```python
from build123d import *

# Parameters (mm, degrees)
CUT_EXTRUDE1_DEPTH = 2


# Read off the part's stored shape, not the designer's step: M6x1.0 Machine Threads Stud1
with BuildPart() as part:
    # Sketch1 → Revolve1 (revolve)
    with BuildSketch(Plane.XY, mode=Mode.PRIVATE) as revolve1_sk:
        with BuildLine():
            Line((0, -16.59536458), (0, 2.796940265))
            Line((0, 2.796940265), (3, 2.796940265))
            ThreePointArc((3, 2.796940265), (6, -2.399212157), (3, -7.59536458))
            Line((3, -7.59536458), (3, -16.59536458))
            Line((3, -16.59536458), (0, -16.59536458))
        make_face()
    revolve(revolve1_sk.sketch.rotate(Axis((0, -16.59536458, 0), (0, 1, 0)), 90), axis=Axis((0, -16.59536458, 0), (0, 1, 0)))

    # Sketch4 → Cut-Extrude1 (cut)
    with BuildSketch(Plane(origin=(0, 2.796940265, 0), x_dir=(1, 0, 0), z_dir=(0, 1, 0))):
        Polygon((-2.05, 0), (-1.025, -1.775352078), (1.025, -1.775352078), (2.05, 0), (1.025, 1.775352078), (-1.025, 1.775352078), align=None)
    extrude(amount=-CUT_EXTRUDE1_DEPTH, mode=Mode.SUBTRACT)

    # M6x1.0 Machine Threads Stud1 outline → M6x1.0 Machine Threads Stud1 (revolve, cut)
    with BuildSketch(Plane.XY):
        Polygon((3, -16.04086458), (2.4455, -16.59536458), (3, -16.59536458), align=None)
    revolve(axis=Axis((0, 0, 0), (0, 1, 0)), mode=Mode.SUBTRACT)


solid = part.part
```
Work out the finished part from the listing and answer in its coordinate system (mm). A direction names the side the tool comes from. Coordinates: 2 decimals unless noted, no trailing zeros. Loops run counter-clockwise (first coordinate to the right, second up) from the corner with the lowest first, then second, coordinate; pieces in that order, holes last. Notation, with made-up numbers: (27, 18.5) - (31, 18.5) arc R19 ccw to (31, 38.5) - close; hole circle Ø10 at (40, 87). An arc over 180 degrees is marked (long way). Use a Markdown table: item, result.
Item 1: Find section C-C, the plane y = -13.25. Determine the outline of the cut face in (x, z).
Evaluation:
| item | result |
|---|---|
| outline | circle Ø6 at (0, 0) |
Item 2: Find section D-D, the plane z = 4. Determine the outline of the cut face in (x, y), and give its area (3 significant figures).
Evaluation:
| item | result |
|---|---|
| outline | circle Ø8.94 at (0, -2.4) |
| area | 62.8 mm2 |
Item 3: Given pin 1 Ø0.6 at (x, y) = (0.5, 2) entering from -Z; pin 2 Ø2 at (y, z) = (-14.5, 0) entering from -X; pin 3 Ø1 at (y, z) = (-10, 0.5) entering from +X, each flat-ended and moving along its own axis, determine where each tip first touches the part or whether it passes through.
Evaluation:
| item | result |
|---|---|
| pin 1 | stops at z = -4.35 |
| pin 2 | stops at x = -3 |
| pin 3 | stops at x = 3 |
Item 4: Find section A-A, the plane x = 0. Determine the outline of the cut face in (y, z).
Evaluation:
| item | result |
|---|---|
| outline | (-16.6, -2.45) - (-16.04, -3) - (-7.6, -3) arc R6 ccw to (2.8, -3) - (2.8, -1.78) - (0.8, -1.78) - (0.8, 1.78) - (2.8, 1.78) - (2.8, 3) arc R6 ccw to (-7.6, 3) - (-16.04, 3) - (-16.6, 2.45) - close |
Item 5: Find section B-B, the plane y = 1.25. Determine the outline of the cut face in (x, z) (3 decimals), and give its area (3 significant figures).
Evaluation:
| item | result |
|---|---|
| outline | circle Ø9.525 at (0, 0); hole (-2.05, 0) - (-1.025, -1.775) - (1.025, -1.775) - (2.05, 0) - (1.025, 1.775) - (-1.025, 1.775) - close |
| area | 60.3 mm2 |
Item 6: Consider probe 1 along Y at (x, z) = (-0.75, 1.5); probe 2 along X at (y, z) = (-3, -0.5); probe 3 along X at (y, z) = (-7.5, 1). Determine where each line is inside the solid, lowest interval first. Write a range as from..to.
Evaluation:
| item | result |
|---|---|
| probe 1 | y = -16.6..0.8 |
| probe 2 | x = -5.95..5.95 |
| probe 3 | x = -3..3 |
Item 7: For faces 1 (the flat face through (1.54, 1.81, -0.88)), 2 (the flat face through (0, 2.797, 2)), determine the directions among +Z, -Z, +X, -X, +Y, -Y from which every point of the face is accessible in a straight line to the end or side of a thin tool.
Evaluation:
| item | result |
|---|---|
| face 1 | +Y |
| face 2 | +Z, -Z, +X, -X, +Y |
Item 8: The mould has two halves that part along X. Classify faces 3 (the flat face through (0, -16.595, 0)), 4 (the cylindrical face through (1.15, -11.88, -2.77)), 5 (the flat face through (0, 2, 1.775)): +X half, -X half, draft (parallel to the pull), parting line (faces both ways), or undercut.
Evaluation:
| item | result |
|---|---|
| face 3 | draft |
| face 4 | parting line |
| face 5 | undercut |
